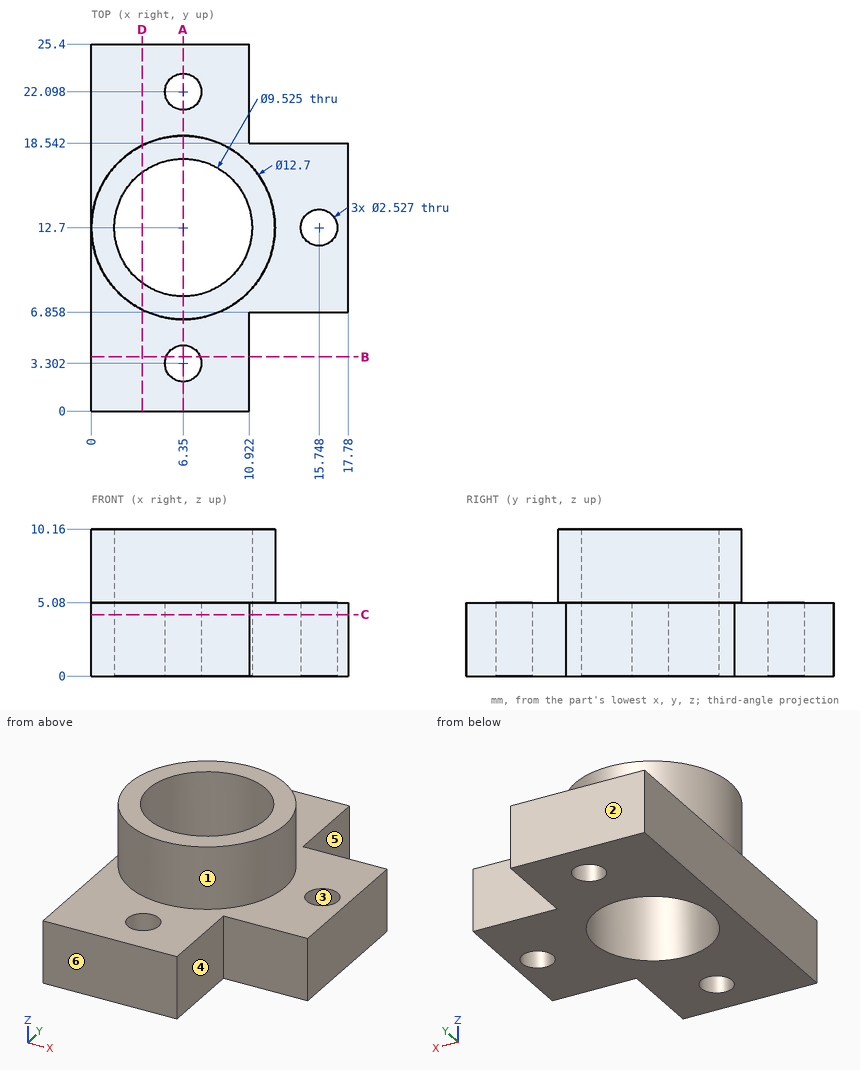
Source: three-view drawing plus pictorial views. Frame: mm from the lowest corner of the part. A direction names the side the tool comes from. Coordinates: 2 decimals unless noted, no trailing zeros. Write each loop counter-clockwise with the first axis right and the second up, starting at its lowest first coordinate (ties: lowest second). Pieces come first, ordered by that corner, then holes. Notation, with made-up numbers: (-12, -27) - (36, -27) arc R16 cw to (36, -21) - close; hole circle Ø9 at (1.5, 83.25). An arc over 180 degrees is marked (long way). Answer as a JSON object with one key per item and string values.
Q1. First-contact query: pin 1 Ø6 at (x, z) = (14.5, 1) entering from -Y; pin 2 Ø6 at (y, z) = (6.5, 5) entering from +X; pin 3 Ø7.5 at (x, y) = (6.35, 12.7) entering from -Z; pin 4 Ø5 at (x, y) = (9, 3) entering from +Z. Flat tips, straight axial feed; report the tip coordinate or a pass-through.
Ans:
{"pin 1": "stops at y = 6.86", "pin 2": "stops at x = 17.78", "pin 3": "passes through", "pin 4": "stops at z = 5.08"}
Q2. Draft query along X for the marked faces 1, 2 and 3. Return one class per face: released by +X, released by -X, zero draft, split by the parting line, or undercut.
Ans:
{"face 1": "split by the parting line", "face 2": "zero draft", "face 3": "undercut"}
Q3. Section query B-B, the plane y = 3.75. Output: boundary loops of the cut face in (x, z), plus the area to 3 significant figures.
Ans:
{"outline": "(0, 0) - (5.17, 0) - (5.17, 5.08) - (0, 5.08) - close; (7.53, 0) - (10.92, 0) - (10.92, 5.08) - (7.53, 5.08) - close", "area": "43.5 mm2"}
Q4. Section query C-C, the plane z = 4.25. State how many separate pieces and enclosed holes the cut face has, plus the area to 3 significant figures.
Ans:
{"separate pieces": "1", "enclosed holes": "4", "area": "271 mm2"}
Q5. Section query D-D, the plane x = 3.5. Output: boundary loops of the cut face in (y, z) (1 decimal).
Ans:
{"outline": "(0, 0) - (8.9, 0) - (8.9, 10.2) - (7, 10.2) - (7, 5.1) - (0, 5.1) - close; (16.5, 0) - (25.4, 0) - (25.4, 5.1) - (18.4, 5.1) - (18.4, 10.2) - (16.5, 10.2) - close"}
Q6. Set-up query: the marked faces 4, 5 and 6. Return all of +Z, -Z, +X, -X, +Y, -Y with unobstructed straight access to the full face (end or side cutting, diameter ignored); none if empty.
Ans:
{"face 4": "+Z, -Z, +X, -Y", "face 5": "+Z, -Z, +X, +Y", "face 6": "+Z, -Z, +X, -X, -Y"}
Q7. Section query A-A, the plane x = 6.35. Output: boundary loops of the cut face in (y, z).
Ans:
{"outline": "(0, 0) - (2.04, 0) - (2.04, 5.08) - (0, 5.08) - close; (4.57, 0) - (7.94, 0) - (7.94, 10.16) - (6.35, 10.16) - (6.35, 5.08) - (4.57, 5.08) - close; (17.46, 0) - (20.83, 0) - (20.83, 5.08) - (19.05, 5.08) - (19.05, 10.16) - (17.46, 10.16) - close; (23.36, 0) - (25.4, 0) - (25.4, 5.08) - (23.36, 5.08) - close"}
Q8. Material intervals for line 1 (Y direction, x = 6.35, z = 1.6); line 2 (X direction, y = 13.5, z = 4.25) (1 decimal); line 3 (X direction, y = 23.25, z = 1) (1 decimal), sorted ascending. Write a range as [from, to].
Ans:
{"line 1": "y = [0, 2.04], [4.57, 7.94], [17.46, 20.83], [23.36, 25.4]", "line 2": "x = [0, 1.7], [11, 14.8], [16.7, 17.8]", "line 3": "x = [0, 5.8], [6.9, 10.9]"}
